from build123d import *

# Parameters (mm, degrees)
BOSS_EXTRUDE2_DEPTH = 234.9999999
CUT_EXTRUDE1_REACH  = 600.452
SKETCH3_R           = 88.9


with BuildPart() as part:
    # Sketch2 → Boss-Extrude2 (new body)
    with BuildSketch(Plane(origin=(0, 0, 0), x_dir=(1, 0, 0), z_dir=(0, 1, 0))):
        Polygon((-263.000000064, 45.001214275), (-263.000000064, -121.405176327), (-150.349364373, -162), (150.349364373, -162), (263.000000064, -121.405176327), (263.000000064, 45.003453118), (261, 45.003453118), (261, -120), (150, -160), (-150, -160), (-261, -120), (-261, 45.001214275), align=None)
    extrude(amount=BOSS_EXTRUDE2_DEPTH)

    # Cut-Extrude1: up to this face of the body (flat: up to its plane)
    cut_extrude1_end = Plane(part.part.faces().sort_by_distance((263.000000064, 117.49999995, 38.200861605))[0])
    # Sketch3 → Cut-Extrude1 (cut, up to the picked face)
    with BuildSketch(Plane.ZY.offset(263.000000064), mode=Mode.PRIVATE) as cut_extrude1_sk1:
        with Locations((24.999999937, -54.80000008)):
            Circle(SKETCH3_R)
    cut_extrude1_tool1 = split(extrude(cut_extrude1_sk1.sketch, amount=-CUT_EXTRUDE1_REACH, mode=Mode.PRIVATE), bisect_by=cut_extrude1_end, keep=Keep.BOTH, mode=Mode.PRIVATE)
    add(cut_extrude1_tool1.solids().sort_by(Axis((-263, -54.8, 25), (1, 0, 0)))[0], mode=Mode.SUBTRACT)


solid = part.part
The model under review builds one solid part; all positions refer to its coordinate system, in mm. A direction names the side the tool comes from. Give positions to 0.01 mm unless a question says otherwise; leave off trailing zeros. Order: outer loops, then holes, each group sorted by start corner. A loop starts at its lowest first (then second) coordinate and runs counter-clockwise, first axis right, second up. Notation, with made-up numbers: M -33,-29 L -1,-29 A29 ccw -1,-4 Z; hole C 61,33 d1. An arc over 180 degrees is marked long. Use one line per item in the form item = value. Start each with the question number.
Item 1: We need section C-C on z = 18. Give the boundary of the cut face in (x, y).
Item 2: The part is to be moulded in two halves that separate along X. For faces 3 (the flat face through (2, 116, 160)), 4 (the flat face through (-1, 0, 161)), 5 (the flat face through (205.886, 115.855, 141.987)), say which applies: pulls with the +X half, pulls with the -X half, needs draft (parallel to the pull), parting line crosses it, or undercut.
Item 3: We need section B-B on y = 133.5. Give the boundary of the cut face in (x, z).
Item 4: Insertion check: pin 1 Ø1 at (x, y) = (-261.5, 140.5) entering from -Z; pin 2 Ø4 at (x, y) = (140.5, 94.5) entering from -Z; pin 3 Ø2 at (x, y) = (-171, 185.5) entering from +Z. Each pin has a flat end and moves straight along its axis. Give the tip position at first contact, or say it passes through.
Item 5: To check wall thickness, follow line 1 along X through (y, z) = (148, 56); line 2 along Z through (x, y) = (-49, 91); line 3 along Z through (x, y) = (-211, 189). State the ranges of each line that lie inside material, in increasing order. Write a range as from..to.
Item 6: We need section D-D on x = -47. Give the boundary of the cut face in (y, z), plus the area to 3 significant figures.
Item 7: We need section A-A on z = -5. Give the boundary of the cut face in (x, y), plus the area to 3 significant figures.
Item 8: For faces 1 (the flat face through (-204.72, 115.85, 140.28)), 2 (the cylindrical face through (-262.014, 34.093, 26.128)), list the 3-axis set-ups (+Z, -Z, +X, -X, +Y, -Y) from which the entire face can be reached by the end or side of a thin tool; tool diameter is ignored.
Completed:
q1.outline = M -263,33.82 L -261,33.82 L -261,235 L -263,235 Z; M 261,33.82 L 263,33.82 L 263,235 L 261,235 Z
q2.face_3 = undercut
q2.face_4 = needs draft
q2.face_5 = pulls with the +X half
q3.outline = M -263,-45 L -261,-45 L -261,120 L -150,160 L 150,160 L 261,120 L 261,-45 L 263,-45 L 263,121.41 L 150.35,162 L -150.35,162 L -263,121.41 Z
q4.pin_1 = -45
q4.pin_2 = 160
q4.pin_3 = 154.92
q5.line_1 = -263..-261, 261..263
q5.line_2 = 160..162
q5.line_3 = 138.02..140.14
q6.outline = M 0,160 L 235,160 L 235,162 L 0,162 Z
q6.area = 470 mm²
q7.outline = M -263,28.89 L -261,28.89 L -261,235 L -263,235 Z; M 261,28.89 L 263,28.89 L 263,235 L 261,235 Z
q7.area = 824 mm²
q8.face_1 = -Z, +Y, -Y
q8.face_2 = +X, -X, -Y
